Geometry: see drawing. Coordinates: mm, zero at the bounding-box minimum. A direction names the side the tool comes from. Round coordinates to 2 decimals unless told otherwise and drop trailing zeros. Loops run counter-clockwise (first coordinate to the right, second up) from the corner with the lowest first, then second, coordinate; pieces in that order, holes last. Notation, with made-up numbers: (-35, 30.5) - (-23, 30.5) arc R26 cw to (-23, 49.5) - close; hole circle Ø10 at (20.25, 51.25). An arc over 180 degrees is marked (long way). Write item = value, one per line. Start each with the question number.
Item 1: Section D-D (z = 40.5). Return loops of the section in (x, y) (3 decimals).
Item 2: Section A-A (x = 32). Return loops of the section in (y, z) (3 decimals).
Item 3: First-contact query: pin 1 (11.5 mm diameter, centred on x = 36, z = 30, fed in from -Y); pin 2 (3 mm diameter, centred on y = 32, z = 10.5, fed in from -X); pin 3 (15 mm diameter, centred on y = 22.5, z = 33.5, fed in from +X). Flat tips, straight axial feed; report the tip coordinate or a pass-through.
Item 4: Line query: line 1 (Z direction, x = 15, y = 53) (3 decimals); line 2 (Z direction, x = 24.55, y = 37.5) (3 decimals); line 3 (Z direction, x = 19, y = 45). Output: solid intervals per line, ascending. Write a range as from..to.
Item 5: Section C-C (z = 25). Return loops of the section in (x, y) (3 decimals), plus the area to 4 significant figures.
Item 6: Section B-B (y = 6.5). Return loops of the section in (x, z) (3 decimals).
Item 7: Access query for the marked faces 1, 2 and 3. Directions: +Z, -Z, +X, -X, +Y, -Y. A direction counts if a zero-diameter tool reaches every point of the face in a straight line with its end or side. Return the directions, or none.
Item 8: Draft query along Z for the marked faces 4, 5 and 6. Return one class per face: pulls with the +Z half, pulls with the -Z half, needs draft (parallel to the pull), parting line crosses it, or undercut.
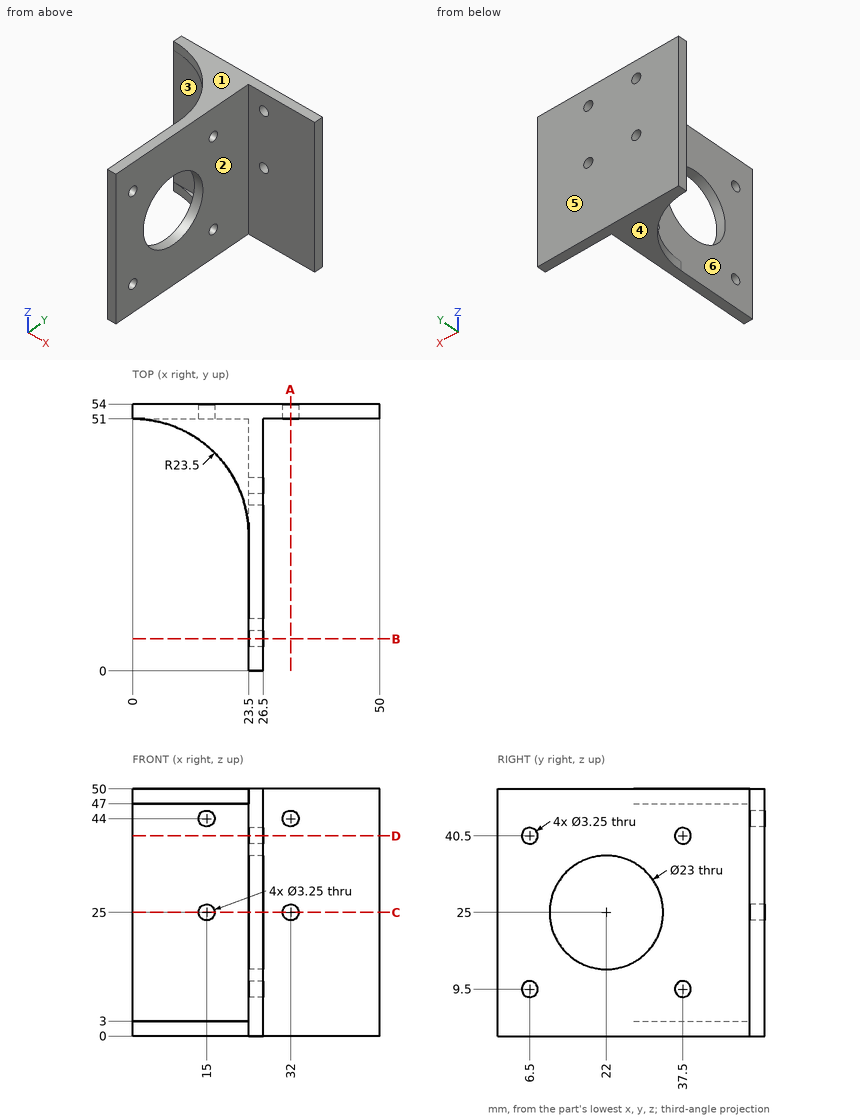
Taken from the geometry:
q1.outline = (0, 51) - (23.5, 51) - (23.5, 39.125) - (26.5, 39.125) - (26.5, 51) - (50, 51) - (50, 54) - (0, 54) - close; (23.5, 0) - (26.5, 0) - (26.5, 4.875) - (23.5, 4.875) - close; (23.5, 8.125) - (26.5, 8.125) - (26.5, 35.875) - (23.5, 35.875) - close
q2.outline = (51, 0) - (54, 0) - (54, 23.375) - (51, 23.375) - close; (51, 26.625) - (54, 26.625) - (54, 42.375) - (51, 42.375) - close; (51, 45.625) - (54, 45.625) - (54, 50) - (51, 50) - close
q3.pin_1 = 51
q3.pin_2 = 23.5
q3.pin_3 = 26.5
q4.line_1 = 0..23.375, 26.625..42.375, 45.625..50
q4.line_2 = 0..7.875, 11.125..38.875, 42.125..50
q4.line_3 = 0..3, 47..50
q5.outline = (0, 51) - (13.375, 51) - (13.375, 54) - (0, 54) - close; (16.625, 51) - (23.5, 51) - (23.5, 33.5) - (26.5, 33.5) - (26.5, 51) - (30.375, 51) - (30.375, 54) - (16.625, 54) - close; (23.5, 0) - (26.5, 0) - (26.5, 10.5) - (23.5, 10.5) - close; (33.625, 51) - (50, 51) - (50, 54) - (33.625, 54) - close
q5.area = 214.5 mm^2
q6.outline = (23.5, 0) - (26.5, 0) - (26.5, 7.875) - (23.5, 7.875) - close; (23.5, 11.125) - (26.5, 11.125) - (26.5, 38.875) - (23.5, 38.875) - close; (23.5, 42.125) - (26.5, 42.125) - (26.5, 50) - (23.5, 50) - close
q7.face_1 = +Z, +X, -X, +Y, -Y
q7.face_2 = +Z, -Z, +X, -Y
q7.face_3 = -X, -Y
q8.face_4 = pulls with the -Z half
q8.face_5 = needs draft
q8.face_6 = undercut
